```python
from build123d import *

# Parameters (mm, degrees)
EXTRUDE_1_DEPTH     = 8
SKETCH_2_R          = 9.85
EXTRUDE_2_DEPTH     = 18.6
SKETCH_3_R          = 8.85
EXTRUDE_3_DEPTH     = 13.6
SKETCH_4_R          = 7.85
EXTRUDE_4_DEPTH     = 11
EXTRUDE_START       = 8
SKETCH_8_R          = 8.85
EXTRUDE_7_DEPTH     = 8
SKETCH_9_R          = 7.35
EXTRUDE_8_DEPTH     = 15
SKETCH_10_R         = 4.5
EXTRUDE_9_DEPTH     = 5
FILLET_1_R          = 10
FILLET_2_R          = 10
FILLET_3_R          = 10
FILLET_4_R          = 10
SKETCH_12_R         = 1
CUT_EXTRUDE_1_DEPTH = 2


with BuildPart() as part:
    # ｽｹｯﾁ1 → ﾎﾞｽ - 押し出し1 (new body)
    with BuildSketch(Plane.XY):
        Polygon((11.05453339, -5.895814181), (10.633191552, 6.625599652), (-0.421341838, 12.521413833), (-11.05453339, 5.895814181), (-10.633191552, -6.625599652), (0.421341838, -12.521413833), align=None)
    extrude(amount=EXTRUDE_1_DEPTH)

    # ｽｹｯﾁ2 → ﾎﾞｽ - 押し出し2 (add)
    with BuildSketch(Plane.XY.offset(8)):
        Circle(SKETCH_2_R)
    extrude(amount=EXTRUDE_2_DEPTH)

    # ｽｹｯﾁ3 → ﾎﾞｽ - 押し出し3 (add)
    with BuildSketch(Plane.XY.offset(26.6)):
        Circle(SKETCH_3_R)
    extrude(amount=EXTRUDE_3_DEPTH)

    # ｽｹｯﾁ4 → ﾎﾞｽ - 押し出し4 (add)
    with BuildSketch(Plane.XY.offset(40.2)):
        Circle(SKETCH_4_R)
    extrude(amount=EXTRUDE_4_DEPTH)

    # ｽｹｯﾁ8 → ﾎﾞｽ - 押し出し7 (add)
    with BuildSketch(Plane(origin=(0, 0, 0), x_dir=(-1, 0, 0), z_dir=(0, 0, -1)).offset(EXTRUDE_START)):
        with Locations(Location((0, 0, 0), (0, 0, 180))):
            Circle(SKETCH_8_R)
    extrude(amount=-EXTRUDE_7_DEPTH)

    # ｽｹｯﾁ9 → ﾎﾞｽ - 押し出し8 (add)
    with BuildSketch(Plane(origin=(0, 0, -8), x_dir=(-1, 0, 0), z_dir=(0, 0, -1))):
        Circle(SKETCH_9_R)
    extrude(amount=EXTRUDE_8_DEPTH)

    # ｽｹｯﾁ10 → ﾎﾞｽ - 押し出し9 (add)
    with BuildSketch(Plane(origin=(0, 0, -23), x_dir=(-1, 0, 0), z_dir=(0, 0, -1))):
        Circle(SKETCH_10_R)
    extrude(amount=EXTRUDE_9_DEPTH)

    # ﾌｨﾚｯﾄ1
    # the kernel refuses this fillet: 10 mm, written as the material it adds along each edge
    with BuildSketch(Plane(origin=(0, 0, 26.6), x_dir=(1, 0, 0), z_dir=(0, -1, 0))) as fillet_1_piece_1:
        with BuildLine():
            CenterArc((18.85, 4.358898944), FILLET_1_R, 180, 25.841932763)
            Line((8.85, 4.358898944), (8.65, 4.358898944))
            Line((8.65, 4.358898944), (8.65, 0))
            Line((8.65, 0), (8.85, -0.2))
            ThreePointArc((8.85, -0.2), (9.35, -0.2), (9.67, -0.087177979))
            Line((9.67, -0.087177979), (9.85, 0))
        make_face()
    revolve(axis=Axis((0, 0, 26.6), (0, 0, 1)))

    # ﾌｨﾚｯﾄ2
    fillet_2_edges = [part.edges().sort_by_distance(p)[0] for p in [
        (-9.85, 0, 26.6),
    ]]
    fillet(fillet_2_edges, radius=FILLET_2_R)

    # ﾌｨﾚｯﾄ3
    # the kernel refuses this fillet: 10 mm, written as the material it adds along each edge
    with BuildSketch(Plane(origin=(0, 0, 40.2), x_dir=(1, 0, 0), z_dir=(0, -1, 0))) as fillet_3_piece_1:
        with BuildLine():
            CenterArc((17.85, 4.358898944), FILLET_3_R, 180, 25.841932763)
            Line((7.85, 4.358898944), (7.65, 4.358898944))
            Line((7.65, 4.358898944), (7.65, 0))
            Line((7.65, 0), (7.85, -0.2))
            ThreePointArc((7.85, -0.2), (8.35, -0.2), (8.67, -0.087177979))
            Line((8.67, -0.087177979), (8.85, 0))
        make_face()
    revolve(axis=Axis((0, 0, 40.2), (0, 0, 1)))

    # ﾌｨﾚｯﾄ4
    fillet_4_edges = [part.edges().sort_by_distance(p)[0] for p in [
        (-8.85, 0, 40.2),
    ]]
    fillet(fillet_4_edges, radius=FILLET_4_R)

    # ｽｹｯﾁ11 → ｶｯﾄ - 回転1 (revolve, cut)
    with BuildSketch(Plane(origin=(0, 0, 0), x_dir=(0, 0, -1), z_dir=(1, 0, 0)), mode=Mode.PRIVATE) as cut_revolve_1_sk:
        with BuildLine():
            Line((25.979017437, 4.5), (28, 4.5))
            Line((28, 4.5), (28, 3.012412215))
            add(Edge.make_bspline(
                [(25.979017437, 4.5), (26.824177567, 4.378307252), (27.771962705, 3.927947166), (28, 3.012412215)],
                knots=[0, 0, 0, 0, 1, 1, 1, 1], degree=3))
        make_face()
    revolve(cut_revolve_1_sk.sketch.rotate(Axis((0, 0, -28), (0, 0, 1)), 90), axis=Axis((0, 0, -28), (0, 0, 1)), mode=Mode.SUBTRACT)

    # ｽｹｯﾁ12 → ｶｯﾄ - 押し出し1 (cut)
    with BuildSketch(Plane.XY.offset(51.2)):
        Circle(SKETCH_12_R)
        with Locations((2.5, 0)):
            Circle(SKETCH_12_R)
        with Locations((5, 0)):
            Circle(SKETCH_12_R)
        with Locations(Location((-5, 0, 0), (0, 0, 180))):
            Circle(SKETCH_12_R)
        with Locations(Location((-2.5, 0, 0), (0, 0, 180))):
            Circle(SKETCH_12_R)
    extrude(amount=-CUT_EXTRUDE_1_DEPTH, mode=Mode.SUBTRACT)


solid = part.part
```
The listing builds one solid part. Answer for the finished solid, in the listing's coordinates (mm). A direction names the side the tool comes from. Give positions to 0.01 mm unless a question says otherwise; leave off trailing zeros. Order: outer loops, then holes, each group sorted by start corner. A loop starts at its lowest first (then second) coordinate and runs counter-clockwise, first axis right, second up. Notation, with made-up numbers: M 42,20.5 L 60,20.5 A23 cw 60,45.5 Z; hole C -6.75,9 d11. An arc over 180 degrees is marked long. Put each result on its own line as item: value. Start each with the question number.
Item 1: Flat-ended cylindrical pins translate along their axes: P1, Ø2, axis at y = 9.5, z = 14, coming from the +X side; P2, Ø2, axis at x = -4, z = 8, coming from the -Y side; P3, Ø1.5, axis at x = -1, y = 6.5, coming from the -Z side. Find the tip coordinate at first contact, or state that the pin passes through.
Item 2: For a pull along X with two mould halves and no side action, classify faces 1 (the face through (0, -2, 51.2)), 2 (the face through (-5.664, 9.255, 3.944)), 3 (the face through (1.593, -7.175, -15.395)), 4 (the face through (-2, 0, 49.2)) as +X half, -X half, draft (parallel to the pull), parting line (faces both ways), or undercut.
Item 3: Which of the six approach directions +Z, -Z, +X, -X, +Y, -Y give full straight-line access (tool end or side, diameter ignored) to faces 5 (the face through (-3, -7, -8)), 6 (the face through (2, 0, 49.2)), 7 (the face through (5.183, 9.532, 3.944))?
Item 4: Find the intervals of material crossed by line 1 along Z through (x, y) = (1.5, 11.25); line 2 along Y through (x, z) = (-2.5, 50.45); line 3 along Y through (x, z) = (5, 50.55), in increasing order.
Item 5: The part is cut by section A-A, the plane z = 4. Determine the outline of the cut face in (x, y), and give its area (3 significant figures).
Item 6: The part is cut by section B-B, the plane y = 11. Determine the outline of the cut face in (x, z).
Item 7: The part is cut by section C-C, the plane z = -20. Determine the outline of the cut face in (x, y).
Answer key:
1. P1: stops at x = 4.98
1. P2: stops at y = -10.7
1. P3: stops at z = -23
2. face 1: draft
2. face 2: -X half
2. face 3: parting line
2. face 4: undercut
3. face 5: -Z
3. face 6: +Z
3. face 7: +Z, -Z, +X, +Y
4. line 1: z = 0 to 8
4. line 2: y = -7.44 to -1, 1 to 7.44
4. line 3: y = -6.05 to -1, 1 to 6.05
5. outline: M -11.05,5.9 L -10.63,-6.63 L 0.42,-12.52 L 11.05,-5.9 L 10.63,6.63 L -0.42,12.52 Z
5. area: 408 mm²
6. outline: M -2.86,0 L 2.43,0 L 2.43,8 L -2.86,8 Z
7. outline: C 0,0 d14.7
